```python
from build123d import *

# Parameters (mm, degrees)
SKETCH_1_R      = 1.6
SKETCH_1_R_2    = 0.599441199
SKETCH_1_R_3    = 0.6
SKETCH_1_R_4    = 0.5
SKETCH_1_R_5    = 0.32499365
SKETCH_1_R_6    = 0.5500127
EXTRUDE_1_DEPTH = 1.399034798


with BuildPart() as part:
    # 草图1 → 凸台-拉伸1 (new body)
    with BuildSketch(Plane.XY.offset(1.399034798)):
        with BuildLine():
            Line((40.06507493, 133.362966726), (110.86507493, 133.362966726))
            ThreePointArc((110.86507493, 133.362966726), (112.694572287, 134.120769344), (113.452374905, 135.950266701))
            Line((113.452374905, 135.950266701), (113.452374905, 172.250266701))
            ThreePointArc((113.452374905, 172.250266701), (112.694572287, 174.079764058), (110.86507493, 174.837566675))
            Line((110.86507493, 174.837566675), (40.06507493, 174.837566675))
            ThreePointArc((40.06507493, 174.837566675), (38.235577573, 174.079764058), (37.477774956, 172.250266701))
            Line((37.477774956, 172.250266701), (37.477774956, 135.950266701))
            ThreePointArc((37.477774956, 135.950266701), (38.235577573, 134.120769344), (40.06507493, 133.362966726))
        make_face()
        with Locations(Location((40.06507493, 172.250266701, 0), (0, 0, 180))):
            Circle(SKETCH_1_R, mode=Mode.SUBTRACT)
        with Locations(Location((51.943103886, 167.132334265, 0), (0, 0, 180))):
            Circle(SKETCH_1_R_2, mode=Mode.SUBTRACT)
        with Locations(Location((54.483108966, 167.132334265, 0), (0, 0, 180))):
            Circle(SKETCH_1_R_2, mode=Mode.SUBTRACT)
        with Locations(Location((57.023114046, 167.132334265, 0), (0, 0, 180))):
            Circle(SKETCH_1_R_2, mode=Mode.SUBTRACT)
        with Locations(Location((51.943103886, 164.592329185, 0), (0, 0, 180))):
            Circle(SKETCH_1_R_2, mode=Mode.SUBTRACT)
        with Locations(Location((54.483108966, 164.592329185, 0), (0, 0, 180))):
            Circle(SKETCH_1_R_2, mode=Mode.SUBTRACT)
        with Locations(Location((57.023114046, 164.592329185, 0), (0, 0, 180))):
            Circle(SKETCH_1_R_2, mode=Mode.SUBTRACT)
        with Locations(Location((59.563119126, 167.132334265, 0), (0, 0, 180))):
            Circle(SKETCH_1_R_2, mode=Mode.SUBTRACT)
        with Locations(Location((62.103124206, 167.132334265, 0), (0, 0, 180))):
            Circle(SKETCH_1_R_2, mode=Mode.SUBTRACT)
        with Locations(Location((64.643129286, 167.132334265, 0), (0, 0, 180))):
            Circle(SKETCH_1_R_2, mode=Mode.SUBTRACT)
        with Locations(Location((59.563119126, 164.592329185, 0), (0, 0, 180))):
            Circle(SKETCH_1_R_2, mode=Mode.SUBTRACT)
        with Locations(Location((62.103124206, 164.592329185, 0), (0, 0, 180))):
            Circle(SKETCH_1_R_2, mode=Mode.SUBTRACT)
        with Locations(Location((64.643129286, 164.592329185, 0), (0, 0, 180))):
            Circle(SKETCH_1_R_2, mode=Mode.SUBTRACT)
        with Locations(Location((67.183134366, 167.132334265, 0), (0, 0, 180))):
            Circle(SKETCH_1_R_2, mode=Mode.SUBTRACT)
        with Locations(Location((69.723139446, 167.132334265, 0), (0, 0, 180))):
            Circle(SKETCH_1_R_2, mode=Mode.SUBTRACT)
        with Locations(Location((67.183134366, 164.592329185, 0), (0, 0, 180))):
            Circle(SKETCH_1_R_2, mode=Mode.SUBTRACT)
        with Locations(Location((69.723139446, 164.592329185, 0), (0, 0, 180))):
            Circle(SKETCH_1_R_2, mode=Mode.SUBTRACT)
        with Locations(Location((51.943103886, 162.052324105, 0), (0, 0, 180))):
            Circle(SKETCH_1_R_2, mode=Mode.SUBTRACT)
        with Locations(Location((54.483108966, 162.052324105, 0), (0, 0, 180))):
            Circle(SKETCH_1_R_2, mode=Mode.SUBTRACT)
        with Locations(Location((57.023114046, 162.052324105, 0), (0, 0, 180))):
            Circle(SKETCH_1_R_2, mode=Mode.SUBTRACT)
        with Locations(Location((59.563119126, 162.052324105, 0), (0, 0, 180))):
            Circle(SKETCH_1_R_2, mode=Mode.SUBTRACT)
        with Locations(Location((62.103124206, 162.052324105, 0), (0, 0, 180))):
            Circle(SKETCH_1_R_2, mode=Mode.SUBTRACT)
        with Locations(Location((64.643129286, 162.052324105, 0), (0, 0, 180))):
            Circle(SKETCH_1_R_2, mode=Mode.SUBTRACT)
        with Locations(Location((67.183134366, 162.052324105, 0), (0, 0, 180))):
            Circle(SKETCH_1_R_2, mode=Mode.SUBTRACT)
        with Locations(Location((69.723139446, 162.052324105, 0), (0, 0, 180))):
            Circle(SKETCH_1_R_2, mode=Mode.SUBTRACT)
        with Locations(Location((65.851363983, 158.524160528, 0), (0, 0, 180))):
            Circle(SKETCH_1_R_3, mode=Mode.SUBTRACT)
        with Locations(Location((65.851363983, 155.984155448, 0), (0, 0, 180))):
            Circle(SKETCH_1_R_3, mode=Mode.SUBTRACT)
        with Locations(Location((68.391369063, 158.524160528, 0), (0, 0, 180))):
            Circle(SKETCH_1_R_3, mode=Mode.SUBTRACT)
        with Locations(Location((68.391369063, 155.984155448, 0), (0, 0, 180))):
            Circle(SKETCH_1_R_3, mode=Mode.SUBTRACT)
        with Locations(Location((93.734188468, 172.334264669, 0), (0, 0, 180))):
            Circle(SKETCH_1_R_4, mode=Mode.SUBTRACT)
        with Locations(Location((101.734188468, 172.334264669, 0), (0, 0, 180))):
            Circle(SKETCH_1_R_4, mode=Mode.SUBTRACT)
        with Locations(Location((110.86507493, 172.250266701, 0), (0, 0, 180))):
            Circle(SKETCH_1_R, mode=Mode.SUBTRACT)
        with Locations(Location((99.949199898, 156.01981204, 0), (0, 0, 180))):
            Circle(SKETCH_1_R_2, mode=Mode.SUBTRACT)
        with Locations(Location((102.489204978, 156.01981204, 0), (0, 0, 180))):
            Circle(SKETCH_1_R_2, mode=Mode.SUBTRACT)
        with Locations(Location((105.029210058, 156.01981204, 0), (0, 0, 180))):
            Circle(SKETCH_1_R_2, mode=Mode.SUBTRACT)
        with Locations(Location((108.662529845, 156.095684531, 0), (0, 0, 180))):
            Circle(SKETCH_1_R_5, mode=Mode.SUBTRACT)
        with Locations(Location((39.168275337, 150.163637287, 0), (0, 0, 180))):
            Circle(SKETCH_1_R_6, mode=Mode.SUBTRACT)
        with Locations(Location((39.168275337, 147.623632207, 0), (0, 0, 180))):
            Circle(SKETCH_1_R_6, mode=Mode.SUBTRACT)
        with Locations(Location((39.168275337, 145.083627127, 0), (0, 0, 180))):
            Circle(SKETCH_1_R_6, mode=Mode.SUBTRACT)
        with Locations(Location((65.851363983, 153.444150368, 0), (0, 0, 180))):
            Circle(SKETCH_1_R_3, mode=Mode.SUBTRACT)
        with Locations(Location((65.851363983, 150.904145288, 0), (0, 0, 180))):
            Circle(SKETCH_1_R_3, mode=Mode.SUBTRACT)
        with Locations(Location((68.391369063, 153.444150368, 0), (0, 0, 180))):
            Circle(SKETCH_1_R_3, mode=Mode.SUBTRACT)
        with Locations(Location((68.391369063, 150.904145288, 0), (0, 0, 180))):
            Circle(SKETCH_1_R_3, mode=Mode.SUBTRACT)
        with Locations(Location((65.851363983, 148.364140208, 0), (0, 0, 180))):
            Circle(SKETCH_1_R_3, mode=Mode.SUBTRACT)
        with Locations(Location((65.851363983, 145.824135128, 0), (0, 0, 180))):
            Circle(SKETCH_1_R_3, mode=Mode.SUBTRACT)
        with Locations(Location((68.391369063, 148.364140208, 0), (0, 0, 180))):
            Circle(SKETCH_1_R_3, mode=Mode.SUBTRACT)
        with Locations(Location((68.391369063, 145.824135128, 0), (0, 0, 180))):
            Circle(SKETCH_1_R_3, mode=Mode.SUBTRACT)
        with Locations(Location((39.168275337, 142.543622047, 0), (0, 0, 180))):
            Circle(SKETCH_1_R_6, mode=Mode.SUBTRACT)
        with Locations(Location((39.168275337, 140.003616967, 0), (0, 0, 180))):
            Circle(SKETCH_1_R_6, mode=Mode.SUBTRACT)
        with Locations(Location((40.06507493, 135.950266701, 0), (0, 0, 180))):
            Circle(SKETCH_1_R, mode=Mode.SUBTRACT)
        with Locations(Location((45.339090678, 135.255270511, 0), (0, 0, 180))):
            Circle(SKETCH_1_R_6, mode=Mode.SUBTRACT)
        with Locations(Location((47.879095758, 135.255270511, 0), (0, 0, 180))):
            Circle(SKETCH_1_R_6, mode=Mode.SUBTRACT)
        with Locations(Location((50.419100838, 135.255270511, 0), (0, 0, 180))):
            Circle(SKETCH_1_R_6, mode=Mode.SUBTRACT)
        with Locations(Location((52.959105918, 135.255270511, 0), (0, 0, 180))):
            Circle(SKETCH_1_R_6, mode=Mode.SUBTRACT)
        with Locations(Location((65.851363983, 143.284130048, 0), (0, 0, 180))):
            Circle(SKETCH_1_R_3, mode=Mode.SUBTRACT)
        with Locations(Location((65.851363983, 140.744124968, 0), (0, 0, 180))):
            Circle(SKETCH_1_R_3, mode=Mode.SUBTRACT)
        with Locations(Location((68.391369063, 143.284130048, 0), (0, 0, 180))):
            Circle(SKETCH_1_R_3, mode=Mode.SUBTRACT)
        with Locations(Location((68.391369063, 140.744124968, 0), (0, 0, 180))):
            Circle(SKETCH_1_R_3, mode=Mode.SUBTRACT)
        with Locations(Location((99.949199898, 153.47980696, 0), (0, 0, 180))):
            Circle(SKETCH_1_R_2, mode=Mode.SUBTRACT)
        with Locations(Location((102.489204978, 153.47980696, 0), (0, 0, 180))):
            Circle(SKETCH_1_R_2, mode=Mode.SUBTRACT)
        with Locations(Location((99.949199898, 150.93980188, 0), (0, 0, 180))):
            Circle(SKETCH_1_R_2, mode=Mode.SUBTRACT)
        with Locations(Location((102.489204978, 150.93980188, 0), (0, 0, 180))):
            Circle(SKETCH_1_R_2, mode=Mode.SUBTRACT)
        with Locations(Location((105.029210058, 153.47980696, 0), (0, 0, 180))):
            Circle(SKETCH_1_R_2, mode=Mode.SUBTRACT)
        with Locations(Location((105.029210058, 150.93980188, 0), (0, 0, 180))):
            Circle(SKETCH_1_R_2, mode=Mode.SUBTRACT)
        with Locations(Location((108.652369825, 150.295836932, 0), (0, 0, 180))):
            Circle(SKETCH_1_R_5, mode=Mode.SUBTRACT)
        with Locations(Location((99.949199898, 148.3997968, 0), (0, 0, 180))):
            Circle(SKETCH_1_R_2, mode=Mode.SUBTRACT)
        with Locations(Location((102.489204978, 148.3997968, 0), (0, 0, 180))):
            Circle(SKETCH_1_R_2, mode=Mode.SUBTRACT)
        with Locations(Location((105.029210058, 148.3997968, 0), (0, 0, 180))):
            Circle(SKETCH_1_R_2, mode=Mode.SUBTRACT)
        with Locations(Location((110.86507493, 135.950266701, 0), (0, 0, 180))):
            Circle(SKETCH_1_R, mode=Mode.SUBTRACT)
        with BuildLine():
            Line((107.612402845, 157.815801372), (108.712402845, 157.815801372))
            ThreePointArc((108.712402845, 157.815801372), (109.012402845, 157.515801372), (108.712402845, 157.215801372))
            Line((108.712402845, 157.215801372), (107.612402845, 157.215801372))
            ThreePointArc((107.612402845, 157.215801372), (107.312402845, 157.515801372), (107.612402845, 157.815801372))
        make_face(mode=Mode.SUBTRACT)
        with BuildLine():
            Line((111.912517145, 157.815801372), (112.712517145, 157.815801372))
            ThreePointArc((112.712517145, 157.815801372), (113.012517145, 157.515801372), (112.712517145, 157.215801372))
            Line((112.712517145, 157.215801372), (111.912517145, 157.215801372))
            ThreePointArc((111.912517145, 157.215801372), (111.612517145, 157.515801372), (111.912517145, 157.815801372))
        make_face(mode=Mode.SUBTRACT)
        with BuildLine():
            Line((107.612402845, 149.175720091), (108.712402845, 149.175720091))
            ThreePointArc((108.712402845, 149.175720091), (109.012402845, 148.875720091), (108.712402845, 148.575720091))
            Line((108.712402845, 148.575720091), (107.612402845, 148.575720091))
            ThreePointArc((107.612402845, 148.575720091), (107.312402845, 148.875720091), (107.612402845, 149.175720091))
        make_face(mode=Mode.SUBTRACT)
        with BuildLine():
            Line((111.912517145, 149.175720091), (112.712517145, 149.175720091))
            ThreePointArc((112.712517145, 149.175720091), (113.012517145, 148.875720091), (112.712517145, 148.575720091))
            Line((112.712517145, 148.575720091), (111.912517145, 148.575720091))
            ThreePointArc((111.912517145, 148.575720091), (111.612517145, 148.875720091), (111.912517145, 149.175720091))
        make_face(mode=Mode.SUBTRACT)
    extrude(amount=-EXTRUDE_1_DEPTH)


solid = part.part
```
Geometry check sheet. Reference: the model listing, model coordinates, mm. Give positions to 0.01 mm unless a question says otherwise; leave off trailing zeros. Write item = value, one per line. Start each with the question number.
1) Gauge pin test, flat ends, axial feed: pin 1 Ø1 at (x, y) = (62.1, 164.59) entering from +Z; pin 2 Ø0.6 at (x, z) = (112, 1) entering from +Y. Record the tip position at first contact, or that the pin passes through.
2) Draft check along Y on faces 1 (the cylindrical face through (38.256, 174.1, 0.709)), 2 (the flat face through (75, 133.363, 1)), 3 (the cylindrical face through (111.073, 170.664, 0.709)), 4 (the flat face through (75, 154, 1.399)). Enter one of: released by +Y, released by -Y, zero draft, split by the parting line, or undercut.
3) Scan lines: L1, parallel to X at y = 151, z = 0.55; L2, parallel to Y at x = 102.5, z = 0.4; L3, parallel to Y at x = 67, z = 0.7. Record each from-to range of solid material in increasing order.
4) Section check A-A (z = 0.95). Count the separate pieces of the cut face and the enclosed holes in it, then the cut area to 3 significant figures.
Geometry check:
q1.pin_1 = through
q1.pin_2 = 174.7
q2.face_1 = released by +Y
q2.face_2 = released by -Y
q2.face_3 = undercut
q2.face_4 = zero draft
q3.L1 = 37.48 to 65.26, 66.44 to 67.8, 68.98 to 99.35, 100.55 to 101.89, 103.09 to 104.43, 105.63 to 113.45
q3.L2 = 133.36 to 147.8, 149 to 150.34, 151.54 to 152.88, 154.08 to 155.42, 156.62 to 174.84
q3.L3 = 133.36 to 161.48, 162.62 to 164.02, 165.16 to 166.56, 167.7 to 174.84
q4.separate_pieces = 1
q4.enclosed_holes = 73
q4.area = 3,040 mm2
